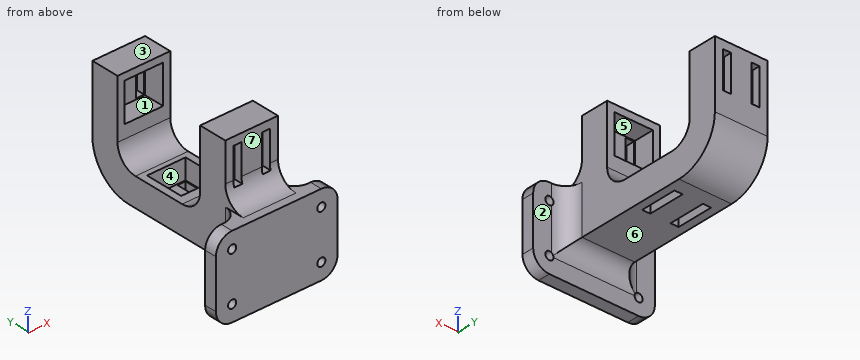
```python
from build123d import *

# Parameters (mm, degrees)
SKETCH1_W            = 13
SKETCH1_H            = 13
SKETCH1_W_2          = 5
SKETCH1_H_2          = 9
BOSS_EXTRUDE1_DEPTH  = 2
SKETCH2_W            = 13
SKETCH2_H            = 13
SKETCH2_W_2          = 9.5
SKETCH2_H_2          = 9.5
BOSS_EXTRUDE2_DEPTH  = 5
SKETCH3_W            = 13
SKETCH3_H            = 13
SKETCH3_W_2          = 5
SKETCH3_H_2          = 9
BOSS_EXTRUDE3_DEPTH  = 2
SKETCH4_W            = 13
SKETCH4_H            = 13
SKETCH4_W_2          = 9.5
SKETCH4_H_2          = 9.5
BOSS_EXTRUDE4_DEPTH  = 5
SKETCH5_W            = 13
SKETCH5_H            = 13
SKETCH5_W_2          = 5
SKETCH5_H_2          = 9
BOSS_EXTRUDE5_DEPTH  = 2
SKETCH6_W            = 13
SKETCH6_H            = 13
SKETCH6_W_2          = 9.5
SKETCH6_H_2          = 9.5
BOSS_EXTRUDE6_DEPTH  = 5
SKETCH7_W            = 13
SKETCH7_H            = 7
BOSS_EXTRUDE7_DEPTH  = 12.5
SKETCH8_W            = 13
SKETCH8_H            = 7
BOSS_EXTRUDE8_DEPTH  = 11.5
BOSS_EXTRUDE9_REACH  = 27.797
SKETCH9_W            = 13
SKETCH9_H            = 7
SKETCH10_W           = 13
SKETCH10_H           = 12
BOSS_EXTRUDE10_DEPTH = 7
SKETCH11_W           = 30
SKETCH11_H           = 20
BOSS_EXTRUDE11_DEPTH = 3
FILLET1_R            = 4
CUT_EXTRUDE1_REACH   = 62.042
SKETCH12_R           = 1
FILLET2_R            = 10
FILLET3_R            = 5


with BuildPart() as part:
    # Sketch1 → Boss-Extrude1 (new body)
    # profile 1 of 2: a face of its own
    with BuildSketch(Plane.XZ.offset(14)):
        with Locations((0, -10)):
            Rectangle(SKETCH1_W, SKETCH1_H)
        Polygon((-4.5, -14.5), (-2.5, -14.5), (2.5, -14.5), (4.5, -14.5), (4.5, -5.5), (2.5, -5.5), (-2.5, -5.5), (-4.5, -5.5), align=None, mode=Mode.SUBTRACT)
    # profile 2 of 2: a face of its own
    with BuildSketch(Plane.XZ.offset(14)):
        with Locations((0, -10)):
            Rectangle(SKETCH1_W_2, SKETCH1_H_2)
    extrude(amount=BOSS_EXTRUDE1_DEPTH)

    # Sketch2 → Boss-Extrude2 (add)
    with BuildSketch(Plane(origin=(0, -14, 0), x_dir=(1, 0, 0), z_dir=(0, 1, 0))):
        with Locations((0, 10)):
            Rectangle(SKETCH2_W, SKETCH2_H)
        with Locations((0, 10)):
            Rectangle(SKETCH2_W_2, SKETCH2_H_2, mode=Mode.SUBTRACT)
    extrude(amount=BOSS_EXTRUDE2_DEPTH)


with BuildPart() as body_2:
    # Sketch3 → Boss-Extrude3 (new body)
    # profile 1 of 2: a face of its own
    with BuildSketch(Plane(origin=(0, 0, -28), x_dir=(-1, 0, 0), z_dir=(0, 0, -1))):
        with Locations((0, 3)):
            Rectangle(SKETCH3_W, SKETCH3_H)
        Polygon((4.5, -1.5), (2.5, -1.5), (-2.5, -1.5), (-4.5, -1.5), (-4.5, 7.5), (-2.5, 7.5), (2.5, 7.5), (4.5, 7.5), align=None, mode=Mode.SUBTRACT)
    # profile 2 of 2: a face of its own
    with BuildSketch(Plane(origin=(0, 0, -28), x_dir=(-1, 0, 0), z_dir=(0, 0, -1))):
        with Locations((0, 3)):
            Rectangle(SKETCH3_W_2, SKETCH3_H_2)
    extrude(amount=BOSS_EXTRUDE3_DEPTH)

    # Sketch4 → Boss-Extrude4 (add)
    with BuildSketch(Plane.XY.offset(-28)):
        with Locations((0, 3)):
            Rectangle(SKETCH4_W, SKETCH4_H)
        with Locations((0, 3)):
            Rectangle(SKETCH4_W_2, SKETCH4_H_2, mode=Mode.SUBTRACT)
    extrude(amount=BOSS_EXTRUDE4_DEPTH)

    # Sketch7 → Boss-Extrude7 (add)
    with BuildSketch(Plane.XZ.offset(3.5)):
        with Locations((0, -26.5)):
            Rectangle(SKETCH7_W, SKETCH7_H)
    extrude(amount=BOSS_EXTRUDE7_DEPTH)

    # Sketch8 → Boss-Extrude8 (add)
    with BuildSketch(Plane(origin=(0, 9.5, 0), x_dir=(1, 0, 0), z_dir=(0, 1, 0))):
        with Locations((0, 26.5)):
            Rectangle(SKETCH8_W, SKETCH8_H)
    extrude(amount=BOSS_EXTRUDE8_DEPTH)

    # Sketch9 → Boss-Extrude9 (add, up to next)
    with BuildSketch(Plane(origin=(0, 0, -16.5), x_dir=(-1, 0, 0), z_dir=(0, 0, -1)), mode=Mode.PRIVATE) as boss_extrude9_sk1:
        with Locations((0, -12.5)):
            Rectangle(SKETCH9_W, SKETCH9_H)
    boss_extrude9_tool1 = extrude(boss_extrude9_sk1.sketch, amount=BOSS_EXTRUDE9_REACH, mode=Mode.PRIVATE) - body_2.part
    # Sketch9 → Boss-Extrude9 (add, up to next)
    with BuildSketch(Plane(origin=(0, 0, -16.5), x_dir=(-1, 0, 0), z_dir=(0, 0, -1)), mode=Mode.PRIVATE) as boss_extrude9_sk2:
        with Locations((0, 17.5)):
            Rectangle(SKETCH9_W, SKETCH9_H)
    boss_extrude9_tool2 = extrude(boss_extrude9_sk2.sketch, amount=BOSS_EXTRUDE9_REACH, mode=Mode.PRIVATE) - body_2.part

    add(part.part)  # Boss-Extrude9 merges part


with BuildPart() as body_3:
    # Sketch5 → Boss-Extrude5 (new body)
    # profile 1 of 2: a face of its own
    with BuildSketch(Plane(origin=(0, 19, 0), x_dir=(1, 0, 0), z_dir=(0, 1, 0))):
        with Locations((0, 10)):
            Rectangle(SKETCH5_W, SKETCH5_H)
        Polygon((-4.5, 14.5), (-2.5, 14.5), (2.5, 14.5), (4.5, 14.5), (4.5, 5.5), (2.5, 5.5), (-2.5, 5.5), (-4.5, 5.5), align=None, mode=Mode.SUBTRACT)
    # profile 2 of 2: a face of its own
    with BuildSketch(Plane(origin=(0, 19, 0), x_dir=(1, 0, 0), z_dir=(0, 1, 0))):
        with Locations((0, 10)):
            Rectangle(SKETCH5_W_2, SKETCH5_H_2)
    extrude(amount=BOSS_EXTRUDE5_DEPTH)

    # Sketch6 → Boss-Extrude6 (add)
    with BuildSketch(Plane.XZ.offset(-19)):
        with Locations((0, -10)):
            Rectangle(SKETCH6_W, SKETCH6_H)
        with Locations((0, -10)):
            Rectangle(SKETCH6_W_2, SKETCH6_H_2, mode=Mode.SUBTRACT)
    extrude(amount=BOSS_EXTRUDE6_DEPTH)


with BuildPart() as body_2_1:
    add(body_2.part)

    add(body_3.part)  # Boss-Extrude9 merges body 3
    add(boss_extrude9_tool1.solids().sort_by_distance((0, -12.5, -16.5))[0])
    add(boss_extrude9_tool2.solids().sort_by_distance((0, 17.5, -16.5))[0])

    # Sketch10 → Boss-Extrude10 (add)
    with BuildSketch(Plane.XZ.offset(16)):
        with Locations((0, -24)):
            Rectangle(SKETCH10_W, SKETCH10_H)
    extrude(amount=BOSS_EXTRUDE10_DEPTH)

    # Sketch11 → Boss-Extrude11 (add)
    with BuildSketch(Plane.XZ.offset(23)):
        with Locations((0, -28)):
            Rectangle(SKETCH11_W, SKETCH11_H)
    extrude(amount=-BOSS_EXTRUDE11_DEPTH)

    # Fillet1
    fillet1_edges = [body_2_1.edges().sort_by_distance(p)[0] for p in [
        (6.5, -20, -24),
        (-6.5, -20, -24),
        (0, -20, -30),
        (-15, -21.5, -18),
        (-15, -21.5, -38),
        (15, -21.5, -18),
        (15, -21.5, -38),
    ]]
    fillet(fillet1_edges, radius=FILLET1_R)

    # Sketch12 → Cut-Extrude1 (cut, up to next)
    with BuildSketch(Plane.XZ.offset(23), mode=Mode.PRIVATE) as cut_extrude1_sk1:
        with Locations(Location((-11, -22, 0), (0, 0, 270))):
            Circle(SKETCH12_R)
    cut_extrude1_tool1 = extrude(cut_extrude1_sk1.sketch, amount=-CUT_EXTRUDE1_REACH, mode=Mode.PRIVATE) & body_2_1.part
    # Sketch12 → Cut-Extrude1 (cut, up to next)
    with BuildSketch(Plane.XZ.offset(23), mode=Mode.PRIVATE) as cut_extrude1_sk2:
        with Locations(Location((11, -22, 0), (0, 0, 270))):
            Circle(SKETCH12_R)
    cut_extrude1_tool2 = extrude(cut_extrude1_sk2.sketch, amount=-CUT_EXTRUDE1_REACH, mode=Mode.PRIVATE) & body_2_1.part
    # Sketch12 → Cut-Extrude1 (cut, up to next)
    with BuildSketch(Plane.XZ.offset(23), mode=Mode.PRIVATE) as cut_extrude1_sk3:
        with Locations(Location((11, -34, 0), (0, 0, 270))):
            Circle(SKETCH12_R)
    cut_extrude1_tool3 = extrude(cut_extrude1_sk3.sketch, amount=-CUT_EXTRUDE1_REACH, mode=Mode.PRIVATE) & body_2_1.part
    # Sketch12 → Cut-Extrude1 (cut, up to next)
    with BuildSketch(Plane.XZ.offset(23), mode=Mode.PRIVATE) as cut_extrude1_sk4:
        with Locations(Location((-11, -34, 0), (0, 0, 270))):
            Circle(SKETCH12_R)
    cut_extrude1_tool4 = extrude(cut_extrude1_sk4.sketch, amount=-CUT_EXTRUDE1_REACH, mode=Mode.PRIVATE) & body_2_1.part
    add(cut_extrude1_tool1.solids().sort_by_distance((-11, -23, -22))[0], mode=Mode.SUBTRACT)
    add(cut_extrude1_tool2.solids().sort_by_distance((11, -23, -22))[0], mode=Mode.SUBTRACT)
    add(cut_extrude1_tool3.solids().sort_by_distance((11, -23, -34))[0], mode=Mode.SUBTRACT)
    add(cut_extrude1_tool4.solids().sort_by_distance((-11, -23, -34))[0], mode=Mode.SUBTRACT)

    # Fillet2
    fillet2_edges = [body_2_1.edges().sort_by_distance(p)[0] for p in [
        (0, 21, -30),
    ]]
    fillet(fillet2_edges, radius=FILLET2_R)

    # Fillet3
    # the kernel refuses this fillet: 5 mm, written as the material it adds along each edge
    with BuildSketch(Plane(origin=(-6.5, 14, -23), x_dir=(0, 0, 1), z_dir=(1, 0, 0)), Plane(origin=(6.5, -9, -23), x_dir=(0, 0, 1), z_dir=(-1, 0, 0))) as fillet3_piece_1:
        with BuildLine():
            CenterArc((FILLET3_R, FILLET3_R), FILLET3_R, 180, 90)
            Line((0, FILLET3_R), (0, 0))
            Line((0, 0), (FILLET3_R, 0))
        make_face()
    extrude(amount=13)
    with BuildSketch(Plane(origin=(-6.5, -16, -18), x_dir=(0, 0, 1), z_dir=(1, 0, 0))) as fillet3_piece_2_section:
        with BuildLine():
            CenterArc((FILLET3_R, FILLET3_R), FILLET3_R, 180, 90)
            Line((0, FILLET3_R), (0, 0))
            Line((0, 0), (FILLET3_R, 0))
        make_face()
    fillet3_piece_2 = extrude(amount=13, mode=Mode.PRIVATE)
    fillet3_piece_2 = split(fillet3_piece_2, bisect_by=Plane(origin=(-5.5, -20.249492121, -14.5), z_dir=(0, 0, -1)), keep=Keep.TOP, mode=Mode.PRIVATE)
    add(fillet3_piece_2)
    with BuildSketch(Plane(origin=(-6.5, -16, -18), x_dir=(0, 0, 1), z_dir=(1, 0, 0))) as fillet3_piece_3_section:
        with BuildLine():
            CenterArc((FILLET3_R, FILLET3_R), FILLET3_R, 180, 90)
            Line((0, FILLET3_R), (0, 0))
            Line((0, 0), (FILLET3_R, 0))
        make_face()
    fillet3_piece_3 = extrude(amount=25.5, mode=Mode.PRIVATE)
    fillet3_piece_3 = split(fillet3_piece_3, bisect_by=Plane(origin=(-4.5, -16.06880959, -14.126748988), z_dir=(-1, 0, 0)), keep=Keep.TOP, mode=Mode.PRIVATE)
    add(fillet3_piece_3)
    with BuildSketch(Plane(origin=(-19, -16, -18), x_dir=(0, 0, 1), z_dir=(1, 0, 0))) as fillet3_piece_4_section:
        with BuildLine():
            CenterArc((FILLET3_R, FILLET3_R), FILLET3_R, 180, 90)
            Line((0, FILLET3_R), (0, 0))
            Line((0, 0), (FILLET3_R, 0))
        make_face()
    fillet3_piece_4 = extrude(amount=38, mode=Mode.PRIVATE)
    fillet3_piece_4 = split(fillet3_piece_4, bisect_by=Plane(origin=(-2.5, -16.06880959, -14.126748988), z_dir=(1, 0, 0)), keep=Keep.TOP, mode=Mode.PRIVATE)
    fillet3_piece_4 = split(fillet3_piece_4, bisect_by=Plane(origin=(2.5, -16.06880959, -14.126748988), z_dir=(-1, 0, 0)), keep=Keep.TOP, mode=Mode.PRIVATE)
    add(fillet3_piece_4)
    with BuildSketch(Plane(origin=(-19, -16, -18), x_dir=(0, 0, 1), z_dir=(1, 0, 0))) as fillet3_piece_5_section:
        with BuildLine():
            CenterArc((FILLET3_R, FILLET3_R), FILLET3_R, 180, 90)
            Line((0, FILLET3_R), (0, 0))
            Line((0, 0), (FILLET3_R, 0))
        make_face()
    fillet3_piece_5 = extrude(amount=25.5, mode=Mode.PRIVATE)
    fillet3_piece_5 = split(fillet3_piece_5, bisect_by=Plane(origin=(4.5, -16.06880959, -14.12674899), z_dir=(1, 0, 0)), keep=Keep.TOP, mode=Mode.PRIVATE)
    add(fillet3_piece_5)


solid = body_2_1.part
```
Could you check a few things on this model? Use its own coordinates, in mm. Face numbers are marked on the shaded views. A direction names the side the tool comes from. Coordinates: 2 decimals unless noted, no trailing zeros. Loops run counter-clockwise (first coordinate to the right, second up) from the corner with the lowest first, then second, coordinate; pieces in that order, holes last. Notation, with made-up numbers: M 86.25,-14 L 134.25,-14 A23 ccw 134.25,20 Z; hole C 72,-19.5 d10. An arc over 180 degrees is marked long. Put each result on its own line as item: value. Start each with the question number.
(1) Suppose I cut it at B-B on x = -5.5. Please give me the cut outline in (y, z), then the cut area to 3 significant figures.
(2) I need wall thicknesses on line 1 (Z direction, x = 11, y = -21); line 2 (X direction, y = -22, z = -34); line 3 (Z direction, x = -5.5, y = 9). Which ranges of each line are inside material? Lowest first, please. Write a range as from..to.
(3) Will these pins go through, and if not, where does the flat tip stop? P1, Ø4, axis at x = 2.5, y = 7, coming from the -Z side; P2, Ø8, axis at x = -4, y = -1, coming from the +Z side; P3, Ø5.5, axis at y = 16, z = -7.5, coming from the +X side.
(4) Suppose I cut it at A-A on z = -17. Please give me the cut outline in (x, y).
(5) For the marked faces 4, 5, 6 and 7, which set-ups out of +Z, -Z, +X, -X, +Y, -Y let a thin tool reach every point of the face, with its end or its side?
(6) Thinking about a two-plate mould opening in Y: for the marked faces 1, 2 and 3, which applies, pulls with the +Y half, pulls with the -Y half, needs draft (parallel to the pull), parting line crosses it, or undercut?
Solutions:
1. outline: M -23,-38 L -20,-38 L -20,-34 A4 cw -16,-30 L 11,-30 A10 ccw 21,-20 L 21,-3.5 L 14,-3.5 L 14,-18 A5 cw 9,-23 L -4,-23 A5 cw -9,-18 L -9,-3.5 L -16,-3.5 L -16,-13 A5 cw -21,-18 L -23,-18 Z
1. area: 638 mm2
2. line 1: z = -38..-35, -33..-23, -21..-18
2. line 2: x = -15..-12, -10..10, 12..15
2. line 3: z = -30..-23
3. P1: stops at z = -30
3. P2: stops at z = -22.9
3. P3: stops at x = 6.5
4. outline: M -6.5,-18 L 6.5,-18 L 6.5,-9 L -6.5,-9 Z; M -6.5,14 L 6.5,14 L 6.5,21 L -6.5,21 Z
5. face 4: +Z
5. face 5: none
5. face 6: -Z, +X, -X, +Y
5. face 7: +Z, +X, -X, -Y
6. face 1: undercut
6. face 2: pulls with the +Y half
6. face 3: needs draft
